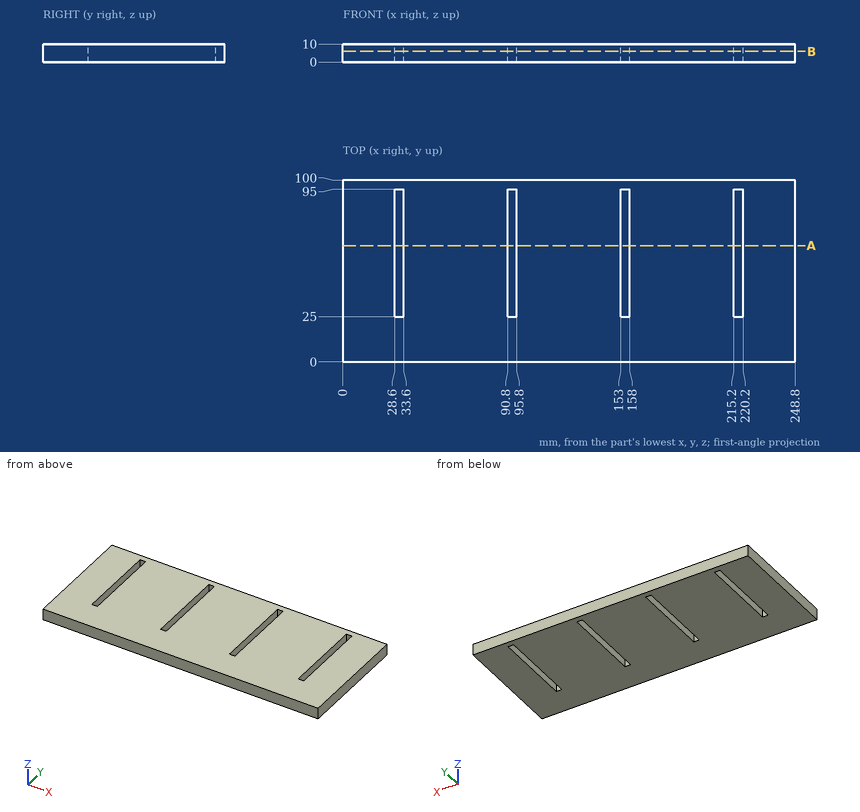
Answer from the drawing. Dimensions are ordinates in mm from the lowest x, y and z of the part. Give positions to 0.01 mm unless a question says otherwise; leave off trailing zeros. Order: outer loops, then holes, each group sorted by start corner. A loop starts at its lowest first (then second) coordinate and runs counter-clockwise, first axis right, second up. Notation, with made-up numbers: (-18, -19.75) -> (28, -19.75) arc R10 ccw to (28, -9.75) -> close; hole circle Ø7 at (35.25, -12). An arc over 180 degrees is marked (long way). Answer as a JSON object with one key per item and string values. Group by question number.
1. A flat-ended cylindrical pin translates along its axis: pin 1 Ø3 at (x, y) = (30.5, 35.5) entering from +Z. Find the tip coordinate at first contact, or state that the pin passes through.
2. Section A-A on y = 64 is taken. Determine the outline of the cut face in (x, z).
3. Section B-B on z = 6 is taken. Determine the outline of the cut face in (x, y).
4. Consider line 1 along X through (y, z) = (28, 3.75); line 2 along Y through (x, z) = (218, 2.75). Determine where each line is inside the solid, lowest interval first. Write a range as [from, to].
Result sheet:
{
 "1": {"pin 1": "passes through"},
 "2": {"outline": "(0, 0) -> (28.6, 0) -> (28.6, 10) -> (0, 10) -> close; (33.6, 0) -> (90.8, 0) -> (90.8, 10) -> (33.6, 10) -> close; (95.8, 0) -> (153, 0) -> (153, 10) -> (95.8, 10) -> close; (158, 0) -> (215.2, 0) -> (215.2, 10) -> (158, 10) -> close; (220.2, 0) -> (248.8, 0) -> (248.8, 10) -> (220.2, 10) -> close"},
 "3": {"outline": "(0, 0) -> (248.8, 0) -> (248.8, 100) -> (0, 100) -> close; hole (28.6, 25) -> (33.6, 25) -> (33.6, 95) -> (28.6, 95) -> close; hole (90.8, 25) -> (95.8, 25) -> (95.8, 95) -> (90.8, 95) -> close; hole (153, 25) -> (158, 25) -> (158, 95) -> (153, 95) -> close; hole (215.2, 25) -> (220.2, 25) -> (220.2, 95) -> (215.2, 95) -> close"},
 "4": {"line 1": "x = [0, 28.6], [33.6, 90.8], [95.8, 153], [158, 215.2], [220.2, 248.8]", "line 2": "y = [0, 25], [95, 100]"}
}
